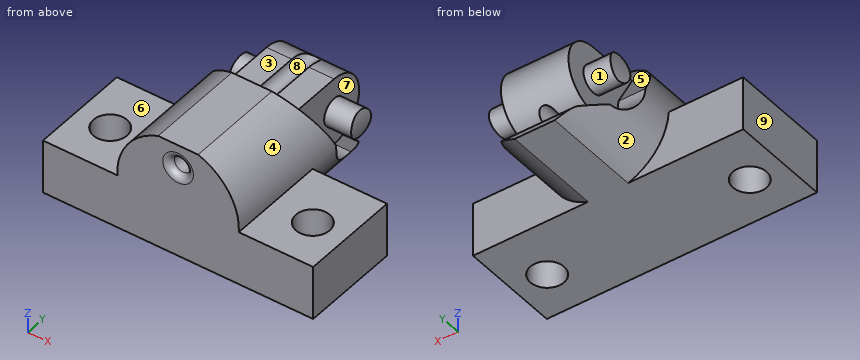
from build123d import *

# Parameters (mm, degrees)
BOSS_EXTRUDE1_DEPTH = 45
SKETCH2_R           = 1.27
CUT_EXTRUDE1_DEPTH  = 51.256
CUT_EXTRUDE2_REACH  = 50.939
SKETCH3_W           = 10
SKETCH3_H           = 10
SKETCH4_R           = 2.049999964
CUT_EXTRUDE3_DEPTH  = 17.5
CUT_EXTRUDE5_START  = -7.95804
SKETCH6_R           = 2
CUT_EXTRUDE5_DEPTH  = 9.6
FILLET3_R           = 1
CUT_EXTRUDE6_START  = 8.64596
SKETCH6_3_R         = 2
CUT_EXTRUDE6_DEPTH  = 6.604
CUT_EXTRUDE7_START  = -14.986
CUT_EXTRUDE7_DEPTH  = 14.986
SKETCH9_W           = 75.785705501
SKETCH9_H           = 55.117400044
CUT_EXTRUDE9_DEPTH  = 51.308
FILLET4_R           = 1
BOSS_EXTRUDE2_START = -9
SKETCH11_W          = 40
SKETCH11_H          = 14.788433541
SKETCH11_R          = 2.5
BOSS_EXTRUDE2_DEPTH = 8


with BuildPart() as part:
    # Sketch1 → Boss-Extrude1 (new body)
    with BuildSketch(Plane(origin=(0, 0, 0), x_dir=(1, 0, 0), z_dir=(0, 1, 0))):
        with BuildLine():
            Line((-2.958039892, 8.5), (2.958039892, 8.5))
            ThreePointArc((2.958039892, 8.5), (9, 0), (2.958039892, -8.5))
            Line((2.958039892, -8.5), (-2.958039892, -8.5))
            ThreePointArc((-2.958039892, -8.5), (-9, 0), (-2.958039892, 8.5))
        make_face()
    extrude(amount=BOSS_EXTRUDE1_DEPTH)

    # Sketch2 → Cut-Extrude1 (cut)
    with BuildSketch(Plane.XZ):
        with Locations(Location((0, -5, 0), (0, 0, 270))):
            Circle(SKETCH2_R)
        with Locations(Location((0, 5, 0), (0, 0, 270))):
            Circle(SKETCH2_R)
    extrude(amount=-CUT_EXTRUDE1_DEPTH, mode=Mode.SUBTRACT)

    # Cut-Extrude2: up to this face of the body (flat: up to its plane)
    cut_extrude2_end = Plane(part.part.faces().sort_by_distance((0, 22.5, 8.5))[0])
    # Sketch3 → Cut-Extrude2 (cut, up to the picked face)
    with BuildSketch(Plane(origin=(0, 0, -8.5), x_dir=(-1, 0, 0), z_dir=(0, 0, -1)), mode=Mode.PRIVATE) as cut_extrude2_sk1:
        with Locations((0, 5)):
            Rectangle(SKETCH3_W, SKETCH3_H)
    cut_extrude2_tool1 = split(extrude(cut_extrude2_sk1.sketch, amount=-CUT_EXTRUDE2_REACH, mode=Mode.PRIVATE), bisect_by=cut_extrude2_end, keep=Keep.BOTH, mode=Mode.PRIVATE)
    add(cut_extrude2_tool1.solids().sort_by(Axis((0, 5, -8.5), (0, 0, 1)))[0], mode=Mode.SUBTRACT)

    # Sketch4 → Cut-Extrude3 (cut, symmetric)
    with BuildSketch(Plane.ZY.offset(-5)):
        with Locations(Location((0, 5, 0), (0, 0, 270))):
            Circle(SKETCH4_R)
        with BuildLine():
            Line((-7.483314774, 10), (-5, 5))
            ThreePointArc((-5, 5), (0, 0), (5, 5))
            Line((5, 5), (8.5, 12.308552788))
            Line((8.5, 12.308552788), (9.857943437, -1.822240199))
            Line((9.857943437, -1.822240199), (-9.857943437, -1.822240199))
            Line((-9.857943437, -1.822240199), (-7.483314774, 10))
        make_face()
    extrude(amount=CUT_EXTRUDE3_DEPTH, both=True, mode=Mode.SUBTRACT)

    # Sketch6 → Cut-Extrude5 (cut)
    with BuildSketch(Plane.ZY.offset(2.958039892).offset(CUT_EXTRUDE5_START)):
        with BuildLine():
            Line((8.5, 30.295597565), (0, 35))
            ThreePointArc((0, 35), (-3.535533906, 36.464466094), (-5, 40))
            Line((-5, 40), (-6.925993812, 43.877868872))
            ThreePointArc((-6.925993812, 43.877868872), (-7.572574331, 44.635904287), (-8.5, 45))
            Line((-8.5, 45), (18.346383487, 50.62633631))
            Line((18.346383487, 50.62633631), (8.5, 30.295597565))
        make_face()
        with Locations((0, 40)):
            Circle(SKETCH6_R, mode=Mode.SUBTRACT)
    extrude(amount=-CUT_EXTRUDE5_DEPTH, mode=Mode.SUBTRACT)

    # Fillet3
    fillet3_edges = [part.edges().sort_by_distance(p)[0] for p in [
        (0, 10, -3.73),
        (0, 10, 6.27),
    ]]
    fillet(fillet3_edges, radius=FILLET3_R)

    # Sketch6<3> → Cut-Extrude6 (cut)
    with BuildSketch(Plane.ZY.offset(2.958039892).offset(CUT_EXTRUDE6_START)):
        with BuildLine():
            Line((8.5, 30.295597565), (0, 35))
            ThreePointArc((0, 35), (-3.535533906, 36.464466094), (-5, 40))
            Line((-5, 40), (-6.925993812, 43.877868872))
            ThreePointArc((-6.925993812, 43.877868872), (-7.572574331, 44.635904287), (-8.5, 45))
            Line((-8.5, 45), (18.346383487, 50.62633631))
            Line((18.346383487, 50.62633631), (8.5, 30.295597565))
        make_face()
        with Locations((0, 40)):
            Circle(SKETCH6_3_R, mode=Mode.SUBTRACT)
    extrude(amount=-CUT_EXTRUDE6_DEPTH, mode=Mode.SUBTRACT)

    # Sketch7 → Cut-Extrude7 (cut)
    with BuildSketch(Plane(origin=(5, 0, 0), x_dir=(0, 0, -1), z_dir=(1, 0, 0)).offset(CUT_EXTRUDE7_START)):
        with BuildLine():
            Line((-5, 40), (-5, 32.23270445))
            Line((-5, 32.23270445), (-8.5, 30.295597565))
            Line((-8.5, 30.295597565), (-10.643597919, 58.76944937))
            Line((-10.643597919, 58.76944937), (18.960626954, 55.630212042))
            Line((18.960626954, 55.630212042), (8.5, 45))
            ThreePointArc((8.5, 45), (7.572574331, 44.635904287), (6.925993812, 43.877868872))
            Line((6.925993812, 43.877868872), (5, 40))
            ThreePointArc((5, 40), (0, 45), (-5, 40))
        make_face()
    extrude(amount=CUT_EXTRUDE7_DEPTH, mode=Mode.SUBTRACT)

    # Sketch9 → Cut-Extrude9 (cut)
    with BuildSketch(Plane.XY.offset(8.5)):
        with Locations((-12.772136987, -12.051535998)):
            Rectangle(SKETCH9_W, SKETCH9_H)
    extrude(amount=-CUT_EXTRUDE9_DEPTH, mode=Mode.SUBTRACT)

    # Fillet4
    fillet4_edges = [part.edges().sort_by_distance(p)[0] for p in [
        (0, 15.507164024, -3.73),
        (0, 15.507164024, 6.27),
    ]]
    fillet(fillet4_edges, radius=FILLET4_R)

    # Sketch11 → Boss-Extrude2 (add)
    with BuildSketch(Plane.XY.offset(8.5).offset(BOSS_EXTRUDE2_START)):
        with Locations((0, 22.901380794)):
            Rectangle(SKETCH11_W, SKETCH11_H)
        with Locations((15, 22.201664168)):
            Circle(SKETCH11_R, mode=Mode.SUBTRACT)
        with Locations((-15, 22.201664168)):
            Circle(SKETCH11_R, mode=Mode.SUBTRACT)
    extrude(amount=-BOSS_EXTRUDE2_DEPTH)


solid = part.part
Could you check a few things on this model? Use its own coordinates, in mm. Face numbers are marked on the shaded views. A direction names the side the tool comes from. Coordinates: 2 decimals unless noted, no trailing zeros. Order: outer loops, then holes, each group sorted by start corner. A loop starts at its lowest first (then second) coordinate and runs counter-clockwise, first axis right, second up. Notation, with made-up numbers: (71, -1) -> (87, -1) arc R10 ccw to (87, 11) -> close; hole circle Ø3 at (-23.75, 38.5). An arc over 180 degrees is marked (long way). One line per question, with ' | ' between items.
Q1. Imagine slicing it at B-B on x = 0. Please give me the cut outline in (y, z), and give its area (3 significant figures).
Return value:
outline: (15.51, -8.5) -> (45, -8.5) arc R2.05 ccw to (43.88, -6.93) -> (42.56, -6.27) -> (30.3, -6.27) -> (30.3, -3.73) -> (43.33, -3.73) arc R5 ccw to (43.33, 3.73) -> (16.51, 3.73) arc R1 ccw to (15.51, 2.73) -> close; (15.51, 7.27) arc R1 ccw to (16.51, 6.27) -> (31.53, 6.27) -> (30.3, 8.5) -> (15.51, 8.5) -> close | area: 352 mm²
Q2. If I drill on L1, parallel to Y at x = -15, z = -3; L2, parallel to Y at x = 10, z = -6.25; L3, parallel to Z at x = 12, y = 30.25, over which ranges is the centre line in solid material (lowest first)?
Return value:
L1: 15.51 to 19.7, 24.7 to 30.3 | L2: 15.51 to 30.3 | L3: -8.5 to -0.5
Q3. Imagine slicing it at C-C on y = 23.5. Please give me the cut outline in (x, z), and give its area (3 significant figures).
Return value:
outline: (-20, -8.5) -> (-17.14, -8.5) -> (-17.14, -0.5) -> (-20, -0.5) -> close; (-12.86, -8.5) -> (12.86, -8.5) -> (12.86, -0.5) -> (8.99, -0.5) arc R9 ccw to (2.96, 8.5) -> (-2.96, 8.5) arc R9 ccw to (-8.99, -0.5) -> (-12.86, -0.5) -> close; (17.14, -8.5) -> (20, -8.5) -> (20, -0.5) -> (17.14, -0.5) -> close; hole circle Ø2.54 at (0, 5) | area: 381 mm²
Q4. I'm going to push flat-ended pins straight in: P1, Ø4, axis at x = 9, z = -6.5, coming from the +Y side; P2, Ø6, axis at x = -15, y = 22.2, coming from the -Z side; P3, Ø1.5, axis at y = 37, z = -1, coming from the +X side; P4, Ø4, axis at x = 4, y = 36.5, coming from the +Z side. Where does each tip first touch, or does it pass through?
Return value:
P1: y = 30.3 | P2: z = -8.5 | P3: x = 5 | P4: z = 5
Q5. Imagine slicing it at A-A on y = 28. Please give me the cut outline in (x, z).
Return value:
outline: (-20, -8.5) -> (20, -8.5) -> (20, -0.5) -> (8.99, -0.5) arc R9 ccw to (2.96, 8.5) -> (-2.96, 8.5) arc R9 ccw to (-8.99, -0.5) -> (-20, -0.5) -> close; hole circle Ø2.54 at (0, 5)
Q6. Thinking about a two-plate mould opening in X: for the marked faces 6, 7, 8 and 9, which applies, pulls with the +X half, pulls with the -X half, needs draft (parallel to the pull), parting line crosses it, or undercut?
Return value:
face 6: needs draft | face 7: pulls with the +X half | face 8: undercut | face 9: pulls with the -X half
Q7. Imagine slicing it at D-D on x = -15. Please give me the cut outline in (y, z).
Return value:
outline: (15.51, -8.5) -> (19.7, -8.5) -> (19.7, -0.5) -> (15.51, -0.5) -> close; (24.7, -8.5) -> (30.3, -8.5) -> (30.3, -0.5) -> (24.7, -0.5) -> close
Q8. On a 3-axis mill with a long thin cutter (end or side, diameter ignored), from which of +Z, -Z, +X, -X, +Y, -Y can I reach the whole of each face in a straight line? I mean the marked faces 1, 2, 3, 4 and 5. Say none if no direction works.
Return value:
face 1: -X | face 2: -X, +Y | face 3: +Z, +X, -X, +Y | face 4: +X, +Y | face 5: +Z
